```python
from build123d import *

# Parameters (mm, degrees)
BOX003_W          = 51.6
BOX003_H          = 0.8
BOX003_DEPTH      = 2
BOX001_W          = 51.6
BOX001_H          = 5
BOX001_DEPTH      = 4
BOX002_W          = 53.2
BOX002_H          = 5.2
BOX002_DEPTH      = 11
BOX008_W          = 3.8
BOX008_H          = 1
BOX008_DEPTH      = 10
CYLINDER002_R     = 1.9
CYLINDER002_DEPTH = 10
CYLINDER004_R     = 1.9
CYLINDER004_DEPTH = 10
ARRAY003_X_COUNT  = 2
ARRAY003_X_PITCH  = 70
BOX006_W          = 80
BOX006_H          = 9.8
BOX006_DEPTH      = 1.5
FILLET003_R       = 3
BOX_W             = 53.2
BOX_H             = 8.2
BOX_DEPTH         = 11


with BuildPart() as bottom_hole_middle_extraction:
    # Box003 → Box003 (new body)
    with BuildSketch(Plane(origin=(0.8, 3.7, 1.5), x_dir=(1, 0, 0), z_dir=(0, 0, 1))):
        with Locations((25.8, 0.4)):
            Rectangle(BOX003_W, BOX003_H)
    extrude(amount=BOX003_DEPTH)


with BuildPart() as bottom_hole_cut:
    # Box001 → Box001 (new body)
    with BuildSketch(Plane(origin=(0.8, 1.6, 1.5), x_dir=(1, 0, 0), z_dir=(0, 0, 1))):
        with Locations((25.8, 2.5)):
            Rectangle(BOX001_W, BOX001_H)
    extrude(amount=BOX001_DEPTH)

    # Cut003003: cut bottom hole middle extraction
    add(bottom_hole_middle_extraction.part, mode=Mode.SUBTRACT)


with BuildPart() as hole_fusion:
    # Box002 → Box002 (new body)
    with BuildSketch(Plane(origin=(0, 1.5, 5.5), x_dir=(1, 0, 0), z_dir=(0, 0, 1))):
        with Locations((26.6, 2.6)):
            Rectangle(BOX002_W, BOX002_H)
    extrude(amount=BOX002_DEPTH)

    # Fusion: union bottom hole cut
    add(bottom_hole_cut.part)


with BuildPart() as obj1:
    # Box008 → Box008 (new body)
    with BuildSketch(Plane(origin=(-1.9, 0, 0), x_dir=(1, 0, 0), z_dir=(0, 0, 1))):
        with Locations((1.9, 0.5)):
            Rectangle(BOX008_W, BOX008_H)
    extrude(amount=BOX008_DEPTH)


with BuildPart() as attach_hole001:
    # Cylinder002 → Cylinder002 (new body)
    with BuildSketch(Plane.XY):
        Circle(CYLINDER002_R)
    extrude(amount=CYLINDER002_DEPTH)


with BuildPart() as attach_hole_array001:
    # Cylinder004 → Cylinder004 (new body)
    with BuildSketch(Plane(origin=(0, 1, 0), x_dir=(1, 0, 0), z_dir=(0, 0, 1))):
        Circle(CYLINDER004_R)
    extrude(amount=CYLINDER004_DEPTH)

    # Fusion002: union obj1, attach hole001
    add(obj1.part)
    add(attach_hole001.part)


with BuildPart() as attach_hole_array001_1:
    # Fusion002 placement: moved
    add(attach_hole_array001.part.moved(Location((5, 4.4, 0))))

    # Array003 X: attach hole array001 ×2


with BuildPart() as attach_hole_array001_2:
    add(attach_hole_array001_1.part)
    with Locations(*[(i * ARRAY003_X_PITCH, 0, 0) for i in range(1, ARRAY003_X_COUNT)]):
        add(attach_hole_array001_1.part)


with BuildPart() as attach_plane_x_dir:
    # Box006 → Box006 (new body)
    with BuildSketch(Plane.XY):
        with Locations((40, 4.9)):
            Rectangle(BOX006_W, BOX006_H)
    extrude(amount=BOX006_DEPTH)

    # Fillet003
    fillet003_edges = [attach_plane_x_dir.edges().sort_by_distance(p)[0] for p in [
        (0, 0, 0.75),
        (0, 9.8, 0.75),
        (80, 0, 0.75),
        (80, 9.8, 0.75),
    ]]
    fillet(fillet003_edges, radius=FILLET003_R)

    # Cut003: cut attach hole array001
    add(attach_hole_array001_2.part, mode=Mode.SUBTRACT)


with BuildPart() as attach_plane_x_dir_1:
    # Cut003 placement: moved
    add(attach_plane_x_dir.part.moved(Location((-13.4, -0.8, 0))))


with BuildPart() as body_cut:
    # Box → Box (new body)
    with BuildSketch(Plane.XY):
        with Locations((26.6, 4.1)):
            Rectangle(BOX_W, BOX_H)
    extrude(amount=BOX_DEPTH)

    # Fusion001: union attach plane x dir
    add(attach_plane_x_dir_1.part)

    # Cut: cut hole fusion
    add(hole_fusion.part, mode=Mode.SUBTRACT)


solid = body_cut.part
```
Read the model definition and answer for the solid it produces. Units are mm, in the model's axes. A direction names the side the tool comes from. Coordinates: 2 decimals unless noted, no trailing zeros. Write each loop counter-clockwise with the first axis right and the second up, starting at its lowest first coordinate (ties: lowest second). Pieces come first, ordered by that corner, then holes. Notation, with made-up numbers: (60, -37) - (109, -37) arc R11 cw to (109, -25) - close; hole circle Ø9 at (65.5, -17). An arc over 180 degrees is marked (long way). Answer as a JSON object with one key per item and string values. Group by question number.
1. Consider L1, parallel to Y at x = 12, z = 2.5; L2, parallel to X at y = 4, z = 1.25; L3, parallel to Y at x = 26, z = 4.5. Determine where each line is inside the solid, lowest interval first. Write a range as [from, to].
2. The mould has two halves that part along X. Classify faces 5 (the flat face through (26, 3, 1.5)), 6 (the flat face through (53.2, 4, 5)), 7 (the flat face through (0, 4, 5)): +X half, -X half, draft (parallel to the pull), parting line (faces both ways), or undercut.
3. A cutting plane is placed at C-C (z = 2.5). Determine the outline of the cut face in (x, y).
4. A cutting plane is placed at A-A (x = -8.4). Determine the outline of the cut face in (y, z), plus the area to 3 significant figures.
5. A cutting plane is placed at B-B (z = 7). Determine the outline of the cut face in (x, y), plus the area to 3 significant figures.
6. A cutting plane is placed at D-D (x = 18). Determine the outline of the cut face in (y, z), plus the area to 3 significant figures.
7. Each of these flat-tipped pins is pushed along its axis until it touches: P1, Ø0.6, axis at x = 18.5, y = 3, coming from the +Z side; P2, Ø5, axis at x = 14, y = 7.5, coming from the -Z side; P3, Ø1.2, axis at x = 39, z = 4, coming from the -Y side; P4, Ø1.2, axis at y = 4.5, z = 4.5, coming from the -X side. Where does it stop, or does it pass through?
8. Which of the six approach directions +Z, -Z, +X, -X, +Y, -Y give full straight-line access (tool end or side, diameter ignored) to faces 1 (the flat face through (26, 1.5, 8)), 2 (the flat face through (26, 8.2, 6)), 3 (the cylindrical face through (61.6, 1.7, 0.7)), 4 (the flat face through (52.4, 4, 4))?
Worked out:
{
 "1": {"L1": "y = [0, 1.6], [3.7, 4.5], [6.6, 8.2]", "L2": "x = [-13.4, -10.3], [-6.5, 59.7], [63.5, 66.6]", "L3": "y = [0, 1.6], [6.6, 8.2]"},
 "2": {"face 5": "undercut", "face 6": "+X half", "face 7": "-X half"},
 "3": {"outline": "(0, 0) - (53.2, 0) - (53.2, 8.2) - (0, 8.2) - close; hole (0.8, 1.6) - (52.4, 1.6) - (52.4, 3.7) - (0.8, 3.7) - close; hole (0.8, 4.5) - (52.4, 4.5) - (52.4, 6.6) - (0.8, 6.6) - close"},
 "4": {"outline": "(-0.8, 0) - (1.7, 0) - (1.7, 1.5) - (-0.8, 1.5) - close; (6.5, 0) - (9, 0) - (9, 1.5) - (6.5, 1.5) - close", "area": "7.50 mm²"},
 "5": {"outline": "(0, 0) - (53.2, 0) - (53.2, 1.5) - (0, 1.5) - close; (0, 6.7) - (53.2, 6.7) - (53.2, 8.2) - (0, 8.2) - close", "area": "160 mm²"},
 "6": {"outline": "(-0.8, 0) - (9, 0) - (9, 1.5) - (8.2, 1.5) - (8.2, 11) - (6.7, 11) - (6.7, 5.5) - (6.6, 5.5) - (6.6, 1.5) - (4.5, 1.5) - (4.5, 3.5) - (3.7, 3.5) - (3.7, 1.5) - (1.6, 1.5) - (1.6, 5.5) - (1.5, 5.5) - (1.5, 11) - (0, 11) - (0, 1.5) - (-0.8, 1.5) - close", "area": "45.6 mm²"},
 "7": {"P1": "stops at z = 1.5", "P2": "stops at z = 0", "P3": "stops at y = 0", "P4": "stops at x = 0"},
 "8": {"face 1": "+Z, +X, -X", "face 2": "+Z, +X, -X, +Y", "face 3": "+Z, -Z", "face 4": "+Z"}
}
